Geometry check sheet. Reference: the model listing, model coordinates, mm. A direction names the side the tool comes from. Round coordinates to 2 decimals unless told otherwise and drop trailing zeros. Write each loop counter-clockwise with the first axis right and the second up, starting at its lowest first coordinate (ties: lowest second). Pieces come first, ordered by that corner, then holes. Notation, with made-up numbers: (-8, -11) - (34, -11) arc R21 cw to (34, 26) - close; hole circle Ø5 at (-19, -25). An arc over 180 degrees is marked (long way). Return JSON: item names as keys, results as strings. Group by question number.
from build123d import *

# Parameters (mm, degrees)
CUT_EXTRUDE_1_DEPTH = 2
FILLET_1_R          = 0.3
CHAMFER_1_SIZE      = 0.3


with BuildPart() as part:
    # Эскиз1 → Повернуть1 (revolve)
    with BuildSketch(Plane(origin=(0, 0, 0), x_dir=(0, 0, -1), z_dir=(1, 0, 0))):
        Polygon((0, 0), (0, 3.5), (4, 3.5), (4, 2), (18, 2), (18, 0), align=None)
    revolve(axis=Axis((0, 0, 0), (0, 0, 1)))

    # Эскиз2 → Вырез-Вытянуть1 (cut)
    with BuildSketch(Plane.XY):
        Polygon((1.732050808, 0), (0.866025404, 1.5), (-0.866025404, 1.5), (-1.732050808, 0), (-0.866025404, -1.5), (0.866025404, -1.5), align=None)
    extrude(amount=-CUT_EXTRUDE_1_DEPTH, mode=Mode.SUBTRACT)

    # Скругление1
    fillet_1_edges = [part.edges().sort_by_distance(p)[0] for p in [
        (0, -2, -4),
    ]]
    fillet(fillet_1_edges, radius=FILLET_1_R)

    # Фаска1
    chamfer_1_edges = [part.edges().sort_by_distance(p)[0] for p in [
        (0, -2, -18),
    ]]
    chamfer(chamfer_1_edges, length=CHAMFER_1_SIZE)


solid = part.part
1. Section check A-A (x = 0). Enter the section's corners in (y, z), and give its area (3 significant figures).
2. Section check C-C (y = 2.5). Enter the section's corners in (x, z), and give its area (3 significant figures).
3. Material ranges on line 1 along Z through (x, y) = (3, 0); line 2 along Y through (x, z) = (-1, -10.25); line 3 along X through (y, z) = (0, -10.25), recorded low to high.
4. Mould release check, pull along Y, two halves, no side actions. Record for faces 4 (the face through (-1.305, -0.74, -0.986)), 5 (the face through (1.341, 3.233, -2.028)), 6 (the face through (0, 0, -18)): pulls with the +Y half, pulls with the -Y half, needs draft (parallel to the pull), parting line crosses it, or undercut.
5. Section check B-B (z = -14). Enter the section's corners in (x, y), and give its area (3 significant figures).
6. Depth check by flat-ended pin: pin 1 Ø2 at (x, z) = (1.5, -6.5) entering from +Y; pin 2 Ø2 at (y, z) = (2, -9) entering from +X; pin 3 Ø1 at (y, z) = (1.5, -16) entering from -X. Enter the tip coordinate at first touch or a pass-through.
7. Tool access check on faces 1 (the face through (0, -2, 0)), 2 (the face through (1.293, -0.76, -0.986)), 3 (the face through (2, 0, -11)). Record the directions out of +Z, -Z, +X, -X, +Y, -Y that give a thin tool (end or side, any length) a straight path to the whole face; none if there is none.
Result sheet:
{
 "1": {"outline": "(-3.5, -4) - (-2.3, -4) arc R0.3 cw to (-2, -4.3) - (-2, -17.7) - (-1.7, -18) - (1.7, -18) - (2, -17.7) - (2, -4.3) arc R0.3 cw to (2.3, -4) - (3.5, -4) - (3.5, 0) - (1.5, 0) - (1.5, -2) - (-1.5, -2) - (-1.5, 0) - (-3.5, 0) - close", "area": "77.9 mm²"},
 "2": {"outline": "(-2.45, -4) - (2.45, -4) - (2.45, 0) - (-2.45, 0) - close", "area": "19.6 mm²"},
 "3": {"line 1": "z = -4 to 0", "line 2": "y = -1.73 to 1.73", "line 3": "x = -2 to 2"},
 "4": {"face 4": "undercut", "face 5": "parting line crosses it", "face 6": "needs draft"},
 "5": {"outline": "circle Ø4 at (0, 0)", "area": "12.6 mm²"},
 "6": {"pin 1": "stops at y = 1.94", "pin 2": "stops at x = 1.73", "pin 3": "stops at x = -1.73"},
 "7": {"face 1": "+Z, +X, -X, +Y, -Y", "face 2": "+Z", "face 3": "-Z"}
}
